Input: part model. Units: mm. Frame: model coordinates. A direction names the side the tool comes from. Coordinates: 2 decimals unless noted, no trailing zeros. Order: outer loops, then holes, each group sorted by start corner. A loop starts at its lowest first (then second) coordinate and runs counter-clockwise, first axis right, second up.
Autodesk Inventor part; units mm, degrees
ref_plane "YZ Plane" through (0, 0, 0) normal (1, 0, 0) x (0, 1, 0)
ref_plane "XZ Plane" through (0, 0, 0) normal (0, 1, 0) x (-1, 0, 0)
ref_plane "XY Plane" through (0, 0, 0) normal (0, 0, 1) x (1, 0, 0)
sketch "Sketch1" plane through (0, 0, 0) normal (0, 1, 0) x (-1, 0, 0)
  line L0 (0, 0) -> (-58, 0)
  line L1 (-58, 0) -> (-58, -41)
  line L2 (-58, -41) -> (0, -41)
  line L3 (0, -41) -> (0, 0)
  dimension "d0" = 58
  dimension "d1" = 41
extrude "Extrusion1" add sketch "Sketch1" along normal blind 4
sketch "Sketch2" plane through (0, 4, 0) normal (0, 1, 0) x (1, 0, 0)
  line L0 (0, 0) -> (58, 0)
  line L1 (58, 0) -> (58, 41)
  line L2 (58, 41) -> (0, 41)
  line L3 (0, 41) -> (0, 0)
  line L4 (4, 37) -> (54, 37)
  line L5 (54, 37) -> (54, 4)
  line L6 (54, 4) -> (4, 4)
  line L7 (4, 4) -> (4, 37)
  line L8 (51, 34) -> (7, 34)
  line L9 (7, 34) -> (7, 7)
  line L10 (7, 7) -> (51, 7)
  line L11 (51, 7) -> (51, 34)
  dimension "d4" = 4
  dimension "d5" = 3
extrude "Extrusion2" add sketch "Sketch2" along normal blind 7 contours L4 L5 L6 L7
sketch "Sketch3" plane through (0, 4, 0) normal (0, 1, 0) x (1, 0, 0)
  line L0 (0, 0) -> (58, 0) construction
  line L1 (58, 0) -> (58, 41) construction
  line L2 (58, 41) -> (0, 41) construction
  line L3 (0, 41) -> (0, 0) construction
  line L4 (54, 37) -> (54, 4) construction
  line L5 (54, 4) -> (4, 4) construction
  line L6 (4, 4) -> (4, 37) construction
  line L7 (4, 37) -> (54, 37) construction
  line L8 (58, 41) -> (0, 41) construction
  line L9 (29, 41) -> (29, 0) construction
  line L10 (0, 41) -> (0, 0) construction
  line L11 (0, 20.5) -> (58, 20.5) construction
  line L12 (58, 0) -> (58, 41) construction
  line L13 (4, 37) -> (4, 4)
  line L14 (4, 8.5) -> (0, 8.5)
  line L15 (0, 8.5) -> (0, 0)
  line L16 (0, 0) -> (9, 0)
  line L17 (0, 0) -> (58, 0)
  line L18 (9, 0) -> (9, 4)
  line L19 (54, 4) -> (4, 4)
  line L20 (9, 4) -> (4, 4)
  line L21 (4, 8.5) -> (4, 4)
  line L22 (17, 0) -> (17, 4)
  line L23 (17, 0) -> (25, 0)
  line L24 (25, 0) -> (25, 4)
  line L25 (25, 4) -> (17, 4)
  line L26 (0, 16.5) -> (4, 16.5)
  line L27 (4, 16.5) -> (4, 20.5)
  line L28 (0, 20.5) -> (0, 16.5)
  line L29 (4, 32.5) -> (0, 32.5)
  line L30 (0, 32.5) -> (0, 41)
  line L31 (0, 41) -> (9, 41)
  line L32 (9, 41) -> (9, 37)
  line L33 (9, 37) -> (4, 37)
  line L34 (4, 32.5) -> (4, 37)
  line L35 (17, 41) -> (17, 37)
  line L36 (17, 41) -> (25, 41)
  line L37 (25, 41) -> (25, 37)
  line L38 (25, 37) -> (17, 37)
  line L39 (0, 24.5) -> (4, 24.5)
  line L40 (4, 24.5) -> (4, 20.5)
  line L41 (0, 20.5) -> (0, 24.5)
  line L42 (58, 41) -> (58, 0) construction
  line L43 (54, 4) -> (54, 37) construction
  line L44 (58, 41) -> (58, 0) construction
  line L45 (54, 37) -> (54, 4)
  line L46 (54, 8.5) -> (58, 8.5)
  line L47 (58, 8.5) -> (58, 0)
  line L48 (58, 0) -> (49, 0)
  line L49 (49, 0) -> (49, 4)
  line L50 (49, 4) -> (54, 4)
  line L51 (54, 8.5) -> (54, 4)
  line L52 (41, 0) -> (41, 4)
  line L53 (41, 0) -> (33, 0)
  line L54 (33, 0) -> (33, 4)
  line L55 (33, 4) -> (41, 4)
  line L56 (58, 16.5) -> (54, 16.5)
  line L57 (54, 16.5) -> (54, 20.5)
  line L58 (58, 20.5) -> (58, 16.5)
  line L59 (41, 41) -> (33, 41)
  line L60 (33, 41) -> (33, 37)
  line L61 (33, 37) -> (41, 37)
  line L62 (54, 32.5) -> (54, 37)
  line L63 (54, 24.5) -> (54, 20.5)
  line L64 (54, 32.5) -> (58, 32.5)
  line L65 (58, 32.5) -> (58, 41)
  line L66 (58, 24.5) -> (54, 24.5)
  line L67 (58, 20.5) -> (58, 24.5)
  line L68 (49, 41) -> (49, 37)
  line L69 (49, 37) -> (54, 37)
  line L70 (58, 41) -> (49, 41)
  line L71 (41, 41) -> (41, 37)
  dimension "d8" = 8
  dimension "d9" = 8
  dimension "d10" = 4
  dimension "d13" = 4
  dimension "d14" = 8
extrude "Extrusion3" cut sketch "Sketch3" against normal up to surface (4 mm away) contours L45 L69 L68 L70 L65 L64 | L45 L66 L67 L58 L56 | L13 L19 L18 L16 L15 L14 | L13 L26 L28 L41 L39 | L13 L29 L30 L31 L32 L33 | L19 L24 L17 L22 | L19 L52 L17 L54 | L19 L45 L46 L47 L17 L49 | L36 L37 L38 L35 | L71 L61 L60 L59
properties part number "bottom" material "PBT Plastic Black"
Item 1: Access query for faces 4 (the face through (49, 2, -2)), 5 (the face through (56, 4, -12)), 6 (the face through (29, 7, -7)), 7 (the face through (13, 4, -39)), 8 (the face through (2, 4, -12)). Directions: +Z, -Z, +X, -X, +Y, -Y. A direction counts if a zero-diameter tool reaches every point of the face in a straight line with its end or side. Return the directions, or none.
Response values:
face 4: +Z, +X, +Y, -Y
face 5: +Z, -Z, +X, +Y
face 6: +Y
face 7: -Z, +X, -X, +Y
face 8: +Z, -Z, -X, +Y
Item 2: Cut plane A-A on x = 18. Return loops of the section in (y, z).
Response values:
outline: (0, -37) - (11, -37) - (11, -34) - (4, -34) - (4, -7) - (11, -7) - (11, -4) - (0, -4) - close
Item 3: Pin query (flat end, axial travel): pin 1 Ø2 at (y, z) = (1, -1) entering from +X; pin 2 Ø3 at (x, y) = (8.5, 6.5) entering from -Z; pin 3 Ø2 at (y, z) = (7, -19.5) entering from -X. Return the tip coordinate at first contact, or that it passes through.
Response values:
pin 1: stops at x = 49
pin 2: stops at z = -37
pin 3: stops at x = 4
Item 4: Cut plane B-B on y = 9. Return loops of the section in (x, z), then the cut area to 3 significant figures.
Response values:
outline: (4, -37) - (54, -37) - (54, -4) - (4, -4) - close; hole (7, -34) - (51, -34) - (51, -7) - (7, -7) - close
area: 462 mm2
Item 5: Cut plane D-D on x = 29. Return loops of the section in (y, z), then the cut area to 3 significant figures.
Response values:
outline: (0, -41) - (4, -41) - (4, -37) - (11, -37) - (11, -34) - (4, -34) - (4, -7) - (11, -7) - (11, -4) - (4, -4) - (4, 0) - (0, 0) - close
area: 206 mm2
Item 6: Ray query, probe 1 along Z at (x, y) = (31, 5.5); probe 2 along X at (y, z) = (5, -19.5); probe 3 along Z at (x, y) = (3.5, 1.5). Return the intervals inside material, ascending.
Response values:
probe 1: z = -37 to -34, -7 to -4
probe 2: x = 4 to 7, 51 to 54
probe 3: z = -32.5 to -24.5, -16.5 to -8.5
Item 7: Cut plane C-C on z = -29. Return loops of the section in (x, y), then the cut area to 3 significant figures.
Response values:
outline: (0, 0) - (58, 0) - (58, 4) - (54, 4) - (54, 11) - (51, 11) - (51, 4) - (7, 4) - (7, 11) - (4, 11) - (4, 4) - (0, 4) - close
area: 274 mm2
Item 8: Draft query along Z for faces 1 (the face through (29, 7, -34)), 2 (the face through (56, 2, -32.5)), 3 (the face through (9, 2, -39)). Return one class per face: pulls with the +Z half, pulls with the -Z half, needs draft (parallel to the pull), parting line crosses it, or undercut.
Response values:
face 1: undercut
face 2: pulls with the -Z half
face 3: needs draft
